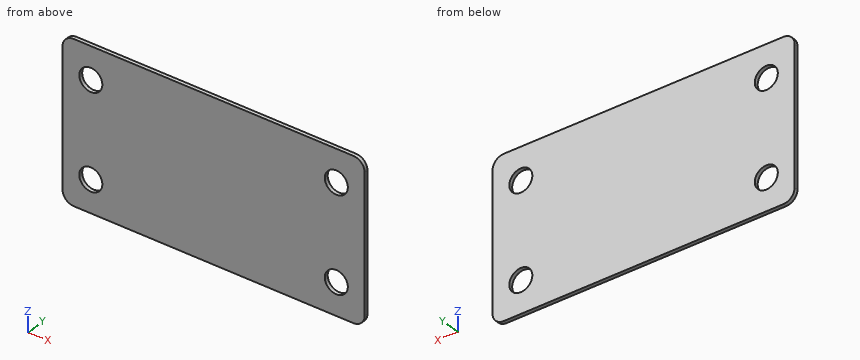
from build123d import *

# Parameters (mm, degrees)
SKETCH_1_W              = 80
SKETCH_1_H              = 42
SM_BASE_FLANGE_1_DEPTH  = 1
FILLET_1_R              = 3
HOLE_WIZARD_6_2_6_2_1_D = 6.1


# Sheet-metal steps are written as plain solids
with BuildPart() as part:
    # Sketch 1 → Базовая кромка1 (new body)
    with BuildSketch(Plane(origin=(0, 0, 0), x_dir=(1, 0, 0), z_dir=(0, 1, 0))):
        Rectangle(SKETCH_1_W, SKETCH_1_H)
    extrude(amount=-SM_BASE_FLANGE_1_DEPTH)

    # Скругление1
    fillet_1_edges = [part.edges().sort_by_distance(p)[0] for p in [
        (40, -0.5, 21),
        (-40, -0.5, 21),
        (-40, -0.5, -21),
        (40, -0.5, -21),
    ]]
    fillet(fillet_1_edges, radius=FILLET_1_R)

    # Диаметр отверстия Ø6.2 (6.2)1 (through all)
    with Locations(Plane(origin=(0, 0, 0), x_dir=(1, 0, 0), z_dir=(0, 1, 0))):
        with Locations((-32.5, 12.5), (-32.5, -12.5), (32.5, -12.5), (32.5, 12.5)):
            Hole(HOLE_WIZARD_6_2_6_2_1_D / 2)


solid = part.part
CAD build for the part. Positions are in the model's coordinates, mm. Round coordinates to 2 decimals unless told otherwise and drop trailing zeros. Write each loop counter-clockwise with the first axis right and the second up, starting at its lowest first coordinate (ties: lowest second). Pieces come first, ordered by that corner, then holes. Notation, with made-up numbers: M 68.25,-10 L 111.25,-10 A10 ccw 111.25,8 Z; hole C 31,57 d11. An arc over 180 degrees is marked long. Put each result on its own line as item: value. Start each with the question number.
1) Pin check, flat tip, straight feed: pin 1 Ø3.5 at (x, z) = (-32.5, -12.5) entering from -Y. Stop position of the tip, or through.
2) Saw through at A-A, the plane x = -32.5. Write the cut outline in (y, z), and give its area (3 significant figures).
3) Drill centre lines: probe 1 along Z at (x, y) = (32.5, -0.65); probe 2 along X at (y, z) = (-0.55, 12.5); probe 3 along X at (y, z) = (-0.2, -13.5). Where is each one in solid material? Low to high. Write a range as [from, to].
4) Saw through at B-B, the plane y = -0.3. Write the cut outline in (x, z).
5) Saw through at C-C, the plane z = -12.5. Write the cut outline in (x, y), and give its area (3 significant figures).
Resolved:
1. pin 1: through
2. outline: M -1,-21 L 0,-21 L 0,-15.55 L -1,-15.55 Z; M -1,-9.45 L 0,-9.45 L 0,9.45 L -1,9.45 Z; M -1,15.55 L 0,15.55 L 0,21 L -1,21 Z
2. area: 29.8 mm²
3. probe 1: [-21, -15.55], [-9.45, 9.45], [15.55, 21]
3. probe 2: [-40, -35.55], [-29.45, 29.45], [35.55, 40]
3. probe 3: [-40, -35.38], [-29.62, 29.62], [35.38, 40]
4. outline: M -40,-18 A3 ccw -37,-21 L 37,-21 A3 ccw 40,-18 L 40,18 A3 ccw 37,21 L -37,21 A3 ccw -40,18 Z; hole C -32.5,-12.5 d6.1; hole C -32.5,12.5 d6.1; hole C 32.5,-12.5 d6.1; hole C 32.5,12.5 d6.1
5. outline: M -40,-1 L -35.55,-1 L -35.55,0 L -40,0 Z; M -29.45,-1 L 29.45,-1 L 29.45,0 L -29.45,0 Z; M 35.55,-1 L 40,-1 L 40,0 L 35.55,0 Z
5. area: 67.8 mm²
